Autodesk Inventor part; units mm, degrees
ref_plane "YZ Plane" through (0, 0, 0) normal (1, 0, 0) x (0, 1, 0)
ref_plane "XZ Plane" through (0, 0, 0) normal (0, 1, 0) x (-1, 0, 0)
ref_plane "XY Plane" through (0, 0, 0) normal (0, 0, 1) x (1, 0, 0)
sketch "Sketch1" plane through (0, 0, 0) normal (0, 1, 0) x (-1, 0, 0)
  line L0 (-2.5, 2.5) -> (2.5, 2.5)
  line L1 (2.5, 2.5) -> (2.5, -2.5)
  line L2 (2.5, -2.5) -> (-2.5, -2.5)
  line L3 (-2.5, -2.5) -> (-2.5, 2.5)
  line L4 (-2.5, 2.5) -> (2.5, -2.5) construction
  line L5 (2.5, 2.5) -> (-2.5, -2.5) construction
  point P0 (0, 0)
  dimension "d0" = 5
  dimension "d1" = 5
extrude "Extrusion1" add sketch "Sketch1" along normal blind 5
shell "Shell1" thickness 1 removed faces 1 at (-0.8333, 5, -0.8333)
sketch "Sketch3" plane through (-2.5, 0, 2.5) normal (0, 0, 1) x (1, 0, 0)
  line L0 (2.5, 9.1674) -> (2.5, 2.1156) construction
  line L1 (1.4995, 9.1674) -> (1.4995, 2.1156)
  line L2 (3.5005, 2.1156) -> (3.5005, 9.1674)
  arc A0 (3.5005, 9.1674) -> (1.4995, 9.1674) centre (2.5, 9.1674) ccw
  arc A1 (1.4995, 2.1156) -> (3.5005, 2.1156) centre (2.5, 2.1156) ccw
  point P0 (2.5, 0)
  point P1 (2.5, 5.6415)
extrude "Extrusion3" cut sketch "Sketch3" against normal through all
sketch "Sketch4" plane through (0, 5, 0) normal (0, 1, 0) x (1, 0, 0)
  point P0 (0, 0)
sketch "Sketch5" plane through (0, 5, 0) normal (0, 1, 0) x (1, 0, 0)
  point P0 (0, 0)
sketch "Sketch6" plane through (0, 5, 0) normal (0, 1, 0) x (1, 0, 0)
  point P0 (0, 0)
sketch "Sketch7" plane through (0, 0, 0) normal (0, -1, 0) x (1, 0, 0)
  point P0 (0, 0)
sketch "Sketch8" plane through (-2.5, 0, -2.5) normal (-1, 0, 0) x (0, 0, 1)
  point P0 (2.5, 0)
properties part number "snapfit_v10"
Check sheet for the modelled part. Datum: model origin and axes. Units: mm. A direction names the side the tool comes from. Give positions to 0.01 mm unless a question says otherwise; leave off trailing zeros. Write each loop counter-clockwise with the first axis right and the second up, starting at its lowest first coordinate (ties: lowest second). Pieces come first, ordered by that corner, then holes.
Item 1: Cross-section at A-A (y = 4.15). Enter the section's corners in (x, z), and give its area (3 significant figures).
Item 2: Draft check along X on faces 4 (the face through (-0.022, 1.115, 2.007)), 5 (the face through (-2.5, 2, 0)), 6 (the face through (2, 5, 0)). Enter one of: released by +X, released by -X, zero draft, split by the parting line, or undercut.
Item 3: Scan lines: L1, parallel to X at y = 2.55, z = -2.1; L2, parallel to X at y = 2.7, z = -0.6. Record each from-to range of solid material in increasing order.
Item 4: Cross-section at D-D (y = 1.95). Enter the section's corners in (x, z), and give its area (3 significant figures).
Item 5: Access from +Z, -Z, +X, -X, +Y, -Y to the whole of each face (thin tool, end or side, straight path). Record for faces 1 (the face through (1.5, 3, 0)), 2 (the face through (-1.15, 1.91, -2.5)), 3 (the face through (-1, 4, 2)).
Item 6: Cross-section at C-C (z = 1.95). Enter the section's corners in (x, y).
Item 7: Cross-section at B-B (x = 1.4). Enter the section's corners in (y, z).
Item 8: Gauge pin test, flat end, axial feed: pin 1 (0.9 mm diameter, centred on x = -0.5, z = -0.5, fed in from +Y). Record the tip position at first contact, or that the pin passes through.
Report:
1. outline: (-2.5, -2.5) - (-1, -2.5) - (-1, -1.5) - (-1.5, -1.5) - (-1.5, 1.5) - (-1, 1.5) - (-1, 2.5) - (-2.5, 2.5) - close; (1, -2.5) - (2.5, -2.5) - (2.5, 2.5) - (1, 2.5) - (1, 1.5) - (1.5, 1.5) - (1.5, -1.5) - (1, -1.5) - close
1. area: 12.0 mm2
2. face 4: undercut
2. face 5: released by -X
2. face 6: zero draft
3. L1: x = -2.5 to -1, 1 to 2.5
3. L2: x = -2.5 to -1.5, 1.5 to 2.5
4. outline: (-2.5, -2.5) - (-0.99, -2.5) - (-0.99, -1.5) - (-1.5, -1.5) - (-1.5, 1.5) - (-0.99, 1.5) - (-0.99, 2.5) - (-2.5, 2.5) - close; (0.99, -2.5) - (2.5, -2.5) - (2.5, 2.5) - (0.99, 2.5) - (0.99, 1.5) - (1.5, 1.5) - (1.5, -1.5) - (0.99, -1.5) - close
4. area: 12.1 mm2
5. face 1: +Y
5. face 2: -Z, +X, -X, +Y, -Y
5. face 3: +Z, -Z, +Y
6. outline: (-2.5, 0) - (2.5, 0) - (2.5, 5) - (1, 5) - (1, 2.12) arc R1 cw to (-1, 2.12) - (-1, 5) - (-2.5, 5) - close
7. outline: (0, -2.5) - (5, -2.5) - (5, -1.5) - (1, -1.5) - (1, 1.5) - (5, 1.5) - (5, 2.5) - (0, 2.5) - close
8. pin 1: stops at y = 1
